Autodesk Inventor part; units mm, degrees
ref_plane "YZ Plane" through (0, 0, 0) normal (1, 0, 0) x (0, 1, 0)
ref_plane "XZ Plane" through (0, 0, 0) normal (0, 1, 0) x (-1, 0, 0)
ref_plane "XY Plane" through (0, 0, 0) normal (0, 0, 1) x (1, 0, 0)
sketch "Sketch1" plane through (0, 0, 0) normal (0, 0, 1) x (1, 0, 0)
  line L0 (-98, 0) -> (-98, 2)
  line L1 (-98, 2) -> (0, 5)
  line L2 (0, 5) -> (0, 0)
  line L3 (0, 0) -> (-98, 0)
  line L4 (0, -25) -> (0, 10)
  point P0 (0, -20)
  dimension "d3" = 2
revolve "Revolution1" add sketch "Sketch1" angle 360 about axis through (0, -10, 0) along (0, 1, 0)
sketch "Sketch2" plane through (0, 0, 0) normal (0, -1, 0) x (1, 0, 0)
  circle A0 centre (0, 0) radius 5
  line L0 (-2.5, -15.4211) -> (2.5, -15.4211)
  line L1 (2.5, -15.4211) -> (2.5, 15.4211)
  line L2 (2.5, 15.4211) -> (-2.5, 15.4211)
  line L3 (-2.5, 15.4211) -> (-2.5, -15.4211)
  line L4 (-2.5, -15.4211) -> (2.5, 15.4211) construction
  line L5 (2.5, -15.4211) -> (-2.5, 15.4211) construction
  point P0 (-2.5, 4.3301)
  point P1 (-2.5, -4.3301)
  point P2 (2.5, -4.3301)
  point P3 (2.5, 4.3301)
  dimension "d8" = 10
  dimension "d9" = 5
extrude "Extrusion1" cut sketch "Sketch2" against normal blind 3 contours L1 A0 L3
properties part number "centrer centrifugal spinner"
For this review, take the finished solid that the model builds, in its own axes (mm). Coordinates: 2 decimals unless noted, no trailing zeros. Write each loop counter-clockwise with the first axis right and the second up, starting at its lowest first coordinate (ties: lowest second). Pieces come first, ordered by that corner, then holes. Notation, with made-up numbers: (21, -0.75) -> (66, -0.75) arc R31 ccw to (66, 29.25) -> close; hole circle Ø9 at (6, -15.5). An arc over 180 degrees is marked (long way). Put each result on its own line as item: value.
Q1. Clearance check with flat-ended pins moving along their axes: pin 1 Ø2.5 at (x, z) = (0.5, 0) entering from -Y; pin 2 Ø2 at (y, z) = (0.5, 71) entering from -X; pin 3 Ø1.5 at (y, z) = (2, -2) entering from +X. State where each tip first meets the part, or that it passes through.
From the geometry:
pin 1: stops at y = 3
pin 2: stops at x = -68.59
pin 3: stops at x = 97.99
Q2. Take a section at A-A, the plane y = 1.2. State the section outline as (x, z) points, then the cut area to 3 significant figures.
From the geometry:
outline: circle Ø196 at (0, 0); hole (-2.5, -4.33) arc R5 ccw to (2.5, -4.33) -> (2.5, 4.33) arc R5 ccw to (-2.5, 4.33) -> close
area: 30,100 mm2
Q3. Wall thickness on L1, parallel to Y at x = -47.5, z = -66.5; L2, parallel to Y at x = -60, z = 76.5; L3, parallel to Z at x = -10, y = 1.2: over which ranges is each line inside the solid? List them lowest first.
From the geometry:
L1: y = 0 to 2.5
L2: y = 0 to 2.02
L3: z = -97.49 to 97.49
Q4. The part is to be moulded in two halves that separate along X. For faces 1 (the flat face through (0, 3, 0)), 2 (the cylindrical face through (-52.684, 1.014, 82.634)), 3 (the flat face through (-20, 0, 1)), say which applies: +X half, -X half, draft (parallel to the pull), parting line (faces both ways), or undercut.
From the geometry:
face 1: undercut
face 2: parting line
face 3: draft
